Design review of the part built by this model. Coordinates are the model's own, in mm. A direction names the side the tool comes from. Coordinates: 2 decimals unless noted, no trailing zeros. Loops run counter-clockwise (first coordinate to the right, second up) from the corner with the lowest first, then second, coordinate; pieces in that order, holes last. Notation, with made-up numbers: (49, 35) - (88, 35) arc R16 ccw to (88, 64) - close; hole circle Ø5 at (-1, 21.5). An arc over 180 degrees is marked (long way). Use one line per item in the form item = value. Start each with the question number.
(1) For L1, parallel to Z at x = 7, y = -1.5; L2, parallel to Z at x = 302, y = -6.5; L3, parallel to Z at x = 179.5, y = -9.5, list the stretches that pass through material, from the lowest coordinate up.
(2) Add section A-A (y = -3.5). State the section outline as (x, z) points (3 decimals), plus the area to 3 significant figures.
(3) Clearance check with flat-ended pins moving along their axes: pin 1 Ø2 at (x, z) = (220, 101.5) entering from +Y; pin 2 Ø5 at (x, y) = (238.5, -6.5) entering from +Z; pin 3 Ø1 at (x, y) = (16.5, -2) entering from -Z; pin 4 Ø4 at (x, y) = (137, -6) entering from -Z. State where each tip first meets the part, or that it passes through.
(4) Tool access review of faces 5 (the face through (-18.719, -6, 231)), 6 (the face through (279.731, -6, 413)), 7 (the face through (32.081, -6, 38)): name each direction out of +Z, -Z, +X, -X, +Y, -Y from which nothing blocks a thin tool from reaching the whole face with its end or side.
(5) Add section C-C (x = 151). State the section outline as (y, z) points, plus the area to 3 significant figures.
(6) The part is to be moulded in two halves that separate along Z. For faces 1 (the face through (158, -6, 400.208)), 2 (the face through (279.731, -6, 38)), 3 (the face through (289.27, -6.26, 26.26)), 4 (the face through (154, -6, 50.958)), say which applies: pulls with the +Z half, pulls with the -Z half, needs draft (parallel to the pull), parting line crosses it, or undercut.
(7) Add section B-B (x = 296.5). State the section outline as (y, z) points.
```python
from build123d import *

# Parameters (mm, degrees)
F0_R     = 15.875
F1_DEPTH = 12.7


with BuildPart() as f1:
    # F0 (on Front) → F1 (new body)
    with BuildSketch(Plane.XZ):
        with BuildLine():
            Line((6.68072, 451.008485), (1.60072, 451.008485))
            ThreePointArc((1.60072, 451.008485), (-12.76769, 445.056895), (-18.71928, 430.688485))
            Line((-18.71928, 430.688485), (-18.71928, 25.558485))
            ThreePointArc((-18.71928, 25.558485), (-11.279792, 7.597973), (6.68072, 0.158485))
            ThreePointArc((6.68072, 0.158485), (24.641232, 7.597973), (32.08072, 25.558485))
            Line((32.08072, 25.558485), (32.08072, 50.958485))
            Line((32.08072, 50.958485), (279.73072, 50.958485))
            Line((279.73072, 50.958485), (279.73072, 25.558485))
            ThreePointArc((279.73072, 25.558485), (287.170208, 7.597973), (305.13072, 0.158485))
            ThreePointArc((305.13072, 0.158485), (323.091232, 7.597973), (330.53072, 25.558485))
            Line((330.53072, 25.558485), (330.53072, 425.608485))
            ThreePointArc((330.53072, 425.608485), (323.091232, 443.568997), (305.13072, 451.008485))
            ThreePointArc((305.13072, 451.008485), (287.170208, 443.568997), (279.73072, 425.608485))
            Line((279.73072, 425.608485), (279.73072, 400.208485))
            Line((279.73072, 400.208485), (32.08072, 400.208485))
            Line((32.08072, 400.208485), (32.08072, 425.608485))
            ThreePointArc((32.08072, 425.608485), (24.641232, 443.568997), (6.68072, 451.008485))
        make_face()
        with Locations((6.68072, 25.558485)):
            Circle(F0_R, mode=Mode.SUBTRACT)
        with Locations((305.13072, 25.558485)):
            Circle(F0_R, mode=Mode.SUBTRACT)
        with Locations((6.68072, 425.608485)):
            Circle(F0_R, mode=Mode.SUBTRACT)
        with Locations((305.13072, 425.608485)):
            Circle(F0_R, mode=Mode.SUBTRACT)
    extrude(amount=F1_DEPTH)


solid = f1.part
```
Computed values:
q1.L1 = 0.16 to 9.69, 41.43 to 409.74, 441.48 to 451.01
q1.L2 = 0.35 to 10, 41.12 to 410.05, 441.17 to 450.81
q1.L3 = 50.96 to 400.21
q2.outline = (-18.719, 25.558) arc R25.4 ccw to (6.681, 0.158) arc R25.4 ccw to (32.081, 25.558) - (32.081, 50.958) - (279.731, 50.958) - (279.731, 25.558) arc R25.4 ccw to (305.131, 0.158) arc R25.4 ccw to (330.531, 25.558) - (330.531, 425.608) arc R25.4 ccw to (305.131, 451.008) arc R25.4 ccw to (279.731, 425.608) - (279.731, 400.208) - (32.081, 400.208) - (32.081, 425.608) arc R25.4 ccw to (6.681, 451.008) - (1.601, 451.008) arc R20.32 ccw to (-18.719, 430.688) - close; hole circle Ø31.75 at (6.681, 25.558); hole circle Ø31.75 at (6.681, 425.608); hole circle Ø31.75 at (305.131, 25.558); hole circle Ø31.75 at (305.131, 425.608)
q2.area = 128,000 mm^2
q3.pin_1 = 0
q3.pin_2 = 400.21
q3.pin_3 = 1.93
q3.pin_4 = 50.96
q4.face_5 = +Z, -Z, -X, +Y, -Y
q4.face_6 = +Z, +Y, -Y
q4.face_7 = -Z, +Y, -Y
q5.outline = (-12.7, 50.96) - (0, 50.96) - (0, 400.21) - (-12.7, 400.21) - close
q5.area = 4,440 mm^2
q6.face_1 = pulls with the +Z half
q6.face_2 = needs draft
q6.face_3 = undercut
q6.face_4 = pulls with the -Z half
q7.outline = (-12.7, 1.67) - (0, 1.67) - (0, 12.23) - (-12.7, 12.23) - close; (-12.7, 38.88) - (0, 38.88) - (0, 412.28) - (-12.7, 412.28) - close; (-12.7, 438.93) - (0, 438.93) - (0, 449.5) - (-12.7, 449.5) - close
